Geometry check sheet. Reference: the model listing, model coordinates, mm. A direction names the side the tool comes from. Round coordinates to 2 decimals unless told otherwise and drop trailing zeros. Loops run counter-clockwise (first coordinate to the right, second up) from the corner with the lowest first, then second, coordinate; pieces in that order, holes last. Notation, with made-up numbers: M -13,-19.5 L 2,-19.5 A31 ccw 2,4.5 Z; hole C 0,-35 d5. An arc over 180 degrees is marked long. Write item = value, one per line.
Autodesk Inventor part; units mm, degrees
ref_plane "YZ Plane" through (0, 0, 0) normal (1, 0, 0) x (0, 1, 0)
ref_plane "XZ Plane" through (0, 0, 0) normal (0, 1, 0) x (-1, 0, 0)
ref_plane "XY Plane" through (0, 0, 0) normal (0, 0, 1) x (1, 0, 0)
sketch "Esquisse1" plane through (0, 0, 0) normal (0, 0, 1) x (1, 0, 0)
  arc A0 (22.8757, 107.3508) -> (1.1243, 107.3508) centre (12, 109) ccw
  arc A1 (9.0085, 2.7745) -> (14.9915, 2.7745) centre (12, 3) ccw
  line L0 (1, 109) -> (9.0085, 2.7745)
  line L1 (23, 109) -> (14.9915, 2.7745)
  point P0 (0, 0)
  dimension "d2" = 22
extrude "Extrusion1" add sketch "Esquisse1" along normal blind 5 contours L1 A1 L0 A0
sketch "Esquisse2" plane through (23, 109, 5) normal (0.9971701, -0.075178, 0) x (0, 0, -1)
  line L0 (5, -109.527) -> (0, -109.527)
  line L1 (2.5, -109.527) -> (1.5, -109.527)
  line L2 (2.5, -109.527) -> (3.5, -109.527)
  line L3 (3.5, -109.527) -> (3.5, -104.527)
  line L4 (3.5, -104.527) -> (1.5, -104.527)
  line L5 (1.5, -104.527) -> (1.5, -109.527)
  point P0 (5, -110.4206)
  dimension "d6" = 1
  dimension "d7" = 1
  dimension "d8" = 5
  dimension "d9" = 2
extrude "Extrusion2" cut sketch "Esquisse2" against normal through all
sketch "Esquisse3" plane through (0, 0, 0) normal (0, 0, -1) x (-1, 0, 0)
  arc A0 (-14.9915, 2.7745) -> (-9.0085, 2.7745) centre (-12, 3) ccw
  arc A1 (-1, 109) -> (-23, 109) centre (-12, 109) ccw
  circle A2 centre (-12, 109) radius 4
  arc A3 (-14.9915, 2.7745) -> (-9.0085, 2.7745) centre (-12, 3) ccw
  line L0 (-12, 0) -> (-12, 2)
  circle A4 centre (-12, 2) radius 1
  line L1 (-14.8284, 2) -> (-9.1716, 2)
  point P0 (0, 0)
  dimension "d13" = 8
  dimension "d24" = 2
  dimension "d25" = 2
  dimension "d26" = 5.6569
extrude "Extrusion3" cut sketch "Esquisse3" against normal through all contours L1 L0 A4 | A4 L1 | L0 L1 A4 | A2
properties part number "Jambe"
(1) Sectioned sample at B-B on z = 2.35. Record the cut outline in (x, y).
Result set:
outline = M 1,109 L 8.82,5.25 L 15.14,4.77 L 23,109 A11 ccw Z; hole C 12,109 d8
(2) Sectioned sample at D-D on x = 6. Record the cut outline in (y, z), then the cut area to 3 significant figures.
Result set:
outline = M 42.68,0 L 118.22,0 L 118.22,5 L 42.68,5 Z
area = 378 mm2
(3) Sectioned sample at C-C on y = 51.5. Record the cut outline in (x, z), then the cut area to 4 significant figures.
Result set:
outline = M 5.34,0 L 18.66,0 L 18.66,5 L 5.34,5 Z
area = 66.65 mm2
(4) Release check for a two-part mould opening along Y. For faces 3 (the cylindrical face through (12, 0, 4)), 4 (the cylindrical face through (12.521, 112.966, 2.465)), 5 (the flat face through (12, 74, 0)) record: released by +Y, released by -Y, zero draft, split by the parting line, or undercut.
Result set:
face_3 = released by -Y
face_4 = undercut
face_5 = zero draft
(5) Sectioned sample at A-A on x = 12. Record the cut outline in (y, z), then the cut area to 3 significant figures.
Result set:
outline = M 0,0 L 1,0 L 1,1.5 L 0,1.5 Z; M 0,3.5 L 1,3.5 L 1,5 L 0,5 Z; M 3,0 L 105,0 L 105,5 L 3,5 L 3,3.5 L 5.01,3.5 L 5.01,1.5 L 3,1.5 Z; M 113,0 L 120,0 L 120,5 L 113,5 Z
area = 544 mm2
(6) Tool access check on faces 1 (the cylindrical face through (12, 0, 1)), 2 (the flat face through (12.026, 5.004, 2.486)). Record the directions out of +Z, -Z, +X, -X, +Y, -Y that give a thin tool (end or side, any length) a straight path to the whole face; none if there is none.
Result set:
face_1 = +Z, -Z, -Y
face_2 = -X, -Y
(7) Depth check by flat-ended pin: pin 1 Ø2 at (x, z) = (13.5, 4) entering from -Y; pin 2 Ø1.5 at (y, z) = (28.5, 3) entering from +X; pin 3 Ø2 at (x, z) = (19.5, 1) entering from +Y. Enter the tip coordinate at first touch or a pass-through.
Result set:
pin_1 = 0.04
pin_2 = 16.99
pin_3 = 117.87
(8) Material ranges on line 1 along Y through (x, z) = (12, 1.1); line 2 along Y through (x, z) = (12, 1.8); line 3 along X through (y, z) = (2, 0.85), recorded low to high. Write a range as from..to.
Result set:
line_1 = 0..1, 3..105, 113..120
line_2 = 5.01..105, 113..120
line_3 = 9.17..11, 13..14.83
